Job drawing, mm, ordinate dimensions from the low corner. One solid piece. Give positions to 0.01 mm unless a question says otherwise; leave off trailing zeros. Loops run counter-clockwise (first coordinate to the right, second up) from the corner with the lowest first, then second, coordinate; pieces in that order, holes last. Notation, with made-up numbers: (27, -5) -> (58, -5) arc R5 cw to (58, 0) -> close; hole circle Ø10 at (49.25, 23). An arc over 180 degrees is marked (long way). Answer as a JSON object with one key per item and string values. Group by question number.
Q1. Band-saw the part on C-C, the plane x = 3.5. Write the cut outline in (y, z), plus the area to 3 significant figures.
Q2. Band-saw the part on B-B, the plane z = 1.15. Write the cut outline in (x, y).
Q3. Band-saw the part on A-A, the plane y = 10. Write the cut outline in (x, z), plus the area to 3 significant figures.
Q4. Wall check: probe 1 along Y at (x, z) = (4, 0.75); probe 2 along Y at (x, z) = (8.5, 1.55); probe 3 along Y at (x, z) = (1.75, 1.1). Give the ranges that are in metal, low to high. Write a range as from..to.
Q5. Band-saw the part on D-D, the plane y = 29.5. Write the cut outline in (x, z), plus the area to 3 significant figures.
Q6. Drop flat-ended pins along their axis: pin 1 (0.6 mm diameter, centred on x = 0.5, z = 1, fed in from +Y); pin 2 (0.6 mm diameter, centred on y = 3, z = 0.5, fed in from -X). Give the stop position or say it passes through.
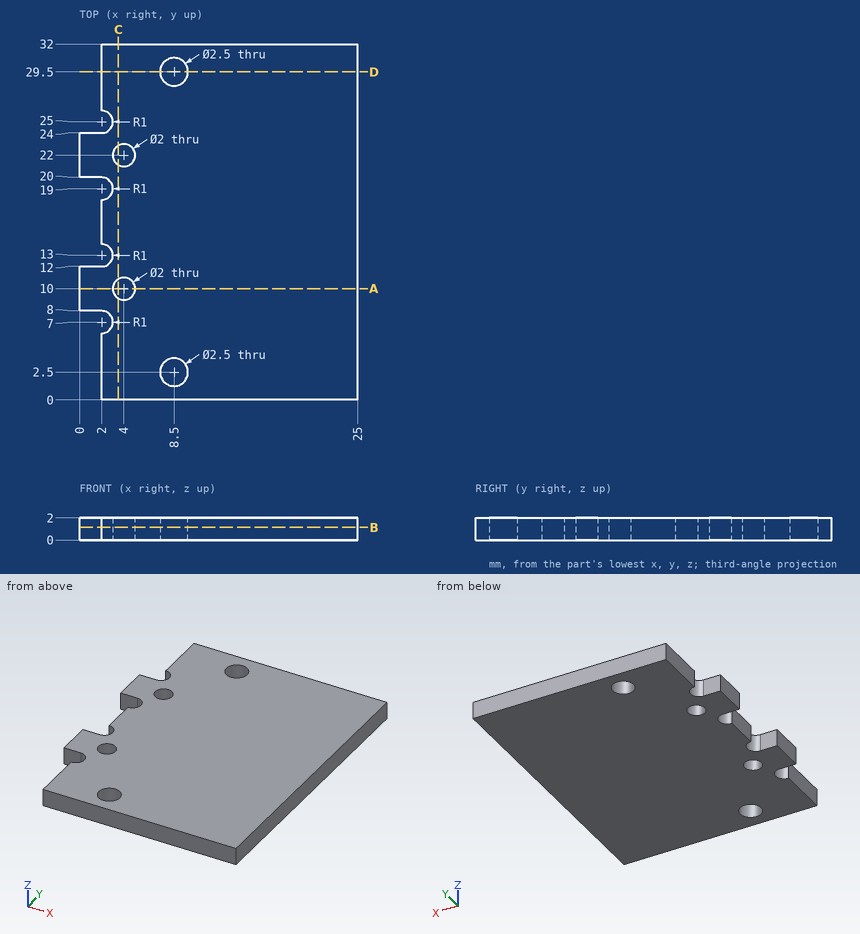
Worked answers:
{
 "1": {"outline": "(0, 0) -> (9.13, 0) -> (9.13, 2) -> (0, 2) -> close; (10.87, 0) -> (21.13, 0) -> (21.13, 2) -> (10.87, 2) -> close; (22.87, 0) -> (32, 0) -> (32, 2) -> (22.87, 2) -> close", "area": "57.1 mm2"},
 "2": {"outline": "(0, 8) -> (2, 8) arc R1 cw to (2, 6) -> (2, 0) -> (25, 0) -> (25, 32) -> (2, 32) -> (2, 26) arc R1 cw to (2, 24) -> (0, 24) -> (0, 20) -> (2, 20) arc R1 cw to (2, 18) -> (2, 14) arc R1 cw to (2, 12) -> (0, 12) -> close; hole circle Ø2 at (4, 10); hole circle Ø2 at (4, 22); hole circle Ø2.5 at (8.5, 2.5); hole circle Ø2.5 at (8.5, 29.5)"},
 "3": {"outline": "(0, 0) -> (3, 0) -> (3, 2) -> (0, 2) -> close; (5, 0) -> (25, 0) -> (25, 2) -> (5, 2) -> close", "area": "46.0 mm2"},
 "4": {"probe 1": "0..9, 11..21, 23..32", "probe 2": "0..1.25, 3.75..28.25, 30.75..32", "probe 3": "8..12, 20..24"},
 "5": {"outline": "(2, 0) -> (7.25, 0) -> (7.25, 2) -> (2, 2) -> close; (9.75, 0) -> (25, 0) -> (25, 2) -> (9.75, 2) -> close", "area": "41.0 mm2"},
 "6": {"pin 1": "y = 24", "pin 2": "x = 2"}
}
